```python
from build123d import *

# Parameters (mm, degrees)
BOSS_EXTRUDE1_DEPTH    = 60
CONVERT_SOLID1_DEPTH   = 60
CONVERT_SOLID1_2_DEPTH = 60
SKETCH7_R              = 2
CUT_EXTRUDE2_DEPTH     = 60
SKETCH10_R             = 4.5
CUT_EXTRUDE3_DEPTH     = 10
SKETCH12_R             = 2.5
CUT_EXTRUDE4_DEPTH     = 10


# Read off the part's stored shape, not the designer's step: Convert-Solid1
with BuildPart() as part:
    # Sketch2 → Boss-Extrude1 (new body)
    with BuildSketch(Plane(origin=(0, 0, 0), x_dir=(0, 0, -1), z_dir=(1, 0, 0))):
        Polygon((0, 70), (0, 0), (50, 0), (50, 4), (4, 4), (4, 70), align=None)
    extrude(amount=BOSS_EXTRUDE1_DEPTH)

    # Convert-Solid1 outline → Convert-Solid1 (cut)
    with BuildSketch(Plane.YZ):
        with BuildLine():
            ThreePointArc((0, -8), (2.343145751, -2.343145751), (8, 0))
            Line((8, 0), (0, 0))
            Line((0, 0), (0, -8))
        make_face()
    extrude(amount=CONVERT_SOLID1_DEPTH, mode=Mode.SUBTRACT)

    # Convert-Solid1 2 outline → Convert-Solid1 2 (add)
    with BuildSketch(Plane.YZ):
        with BuildLine():
            ThreePointArc((4, -8), (5.171572875, -5.171572875), (8, -4))
            Line((8, -4), (4, -4))
            Line((4, -4), (4, -8))
        make_face()
    extrude(amount=CONVERT_SOLID1_2_DEPTH)

    # Sketch7 → Cut-Extrude2 (cut)
    with BuildSketch(Plane(origin=(0, 4, 0), x_dir=(1, 0, 0), z_dir=(0, 1, 0))):
        with Locations(Location((15, 29.476677551, 0), (0, 0, 270))):
            Circle(SKETCH7_R)
    cut_extrude2 = extrude(amount=-CUT_EXTRUDE2_DEPTH, mode=Mode.SUBTRACT)

    # Mirror1: Cut-Extrude2 across plane
    add(cut_extrude2.mirror(Plane.ZY.offset(-30)), mode=Mode.SUBTRACT)

    # Sketch10 → Cut-Extrude3 (cut)
    with BuildSketch(Plane(origin=(0, 0, -4), x_dir=(-1, 0, 0), z_dir=(0, 0, -1))):
        with Locations(Location((-30, 32, 0), (0, 0, 90))):
            Circle(SKETCH10_R)
    extrude(amount=-CUT_EXTRUDE3_DEPTH, mode=Mode.SUBTRACT)

    # Sketch12 → Cut-Extrude4 (cut)
    with BuildSketch(Plane(origin=(0, 0, -4), x_dir=(-1, 0, 0), z_dir=(0, 0, -1))):
        with Locations(Location((-48.499902666, 32.060011256, 0), (0, 0, 90))):
            Circle(SKETCH12_R)
        with Locations(Location((-11.5, 32.060011256, 0), (0, 0, 90))):
            Circle(SKETCH12_R)
    extrude(amount=-CUT_EXTRUDE4_DEPTH, mode=Mode.SUBTRACT)


solid = part.part
```
Work out the finished part from the listing and answer in its coordinate system (mm). A direction names the side the tool comes from. Coordinates: 2 decimals unless noted, no trailing zeros. Loops run counter-clockwise (first coordinate to the right, second up) from the corner with the lowest first, then second, coordinate; pieces in that order, holes last. Notation, with made-up numbers: (-3, 81.25) -> (46, 81.25) arc R22 ccw to (46, 113.25) -> close; hole circle Ø10 at (18.25, 31). An arc over 180 degrees is marked (long way). Answer as CSV lines item,"result".
Q1. Find the intervals of material crossed by probe 1 along X at (y, z) = (32, -2.05); probe 2 along Z at (x, y) = (32.5, 40); probe 3 along Y at (x, z) = (52, -38), in increasing order.
Findings:
probe 1,"x = 0 to 9, 14 to 25.5, 34.5 to 46, 51 to 60"
probe 2,"z = -4 to 0"
probe 3,"y = 0 to 4"
Q2. Each of these flat-tipped pins is pushed along its axis until it touches: pin 1 (5 mm diameter, centred on x = 12, y = 16.5, fed in from -Z); pin 2 (3 mm diameter, centred on x = 48.5, y = 32.06, fed in from +Z); pin 3 (8 mm diameter, centred on x = 29.5, z = -15.5, fed in from +Y). Where does it stop, or does it pass through?
Findings:
pin 1,"stops at z = -4"
pin 2,"passes through"
pin 3,"stops at y = 4"
Q3. For a pull along X with two mould halves and no side action, classify faces 1 (the face through (46.774, 2.028, -28.554)), 2 (the face through (30, 70, -2)), 3 (the face through (0, 19, -3)) as +X half, -X half, draft (parallel to the pull), parting line (faces both ways), or undercut.
Findings:
face 1,"undercut"
face 2,"draft"
face 3,"-X half"
Q4. The part is cut by section B-B on y = 32. Write down the section's boundary in (x, z), and give its area (3 significant figures).
Findings:
outline,"(0, -4) -> (9, -4) -> (9, 0) -> (0, 0) -> close; (14, -4) -> (25.5, -4) -> (25.5, 0) -> (14, 0) -> close; (34.5, -4) -> (46, -4) -> (46, 0) -> (34.5, 0) -> close; (51, -4) -> (60, -4) -> (60, 0) -> (51, 0) -> close"
area,"164 mm²"
Q5. The part is cut by section D-D on z = -3. Write down the section's boundary in (x, y) (3 decimals), and give its area (3 significant figures).
Findings:
outline,"(0, 1.755) -> (60, 1.755) -> (60, 70) -> (0, 70) -> close; hole circle Ø5 at (11.5, 32.06); hole circle Ø9 at (30, 32); hole circle Ø5 at (48.5, 32.06)"
area,"3,990 mm²"
Q6. The part is cut by section A-A on x = 11.5. Write down the section's boundary in (y, z), and give its area (3 significant figures).
Findings:
outline,"(0, -50) -> (4, -50) -> (4, -8) arc R4 cw to (8, -4) -> (29.56, -4) -> (29.56, 0) -> (8, 0) arc R8 ccw to (0, -8) -> close; (34.56, -4) -> (70, -4) -> (70, 0) -> (34.56, 0) -> close"
area,"434 mm²"
Q7. A tool of negligible diameter and unlimited length cuts with its end or side. For faces 4 (the face through (16.686, 2.028, -28.401)), 5 (the face through (30, 4, -29)), from which of +Z, -Z, +X, -X, +Y, -Y can it reach the whole face along a straight path? Write none if from no direction.
Findings:
face 4,"+Y, -Y"
face 5,"-Z, +X, -X, +Y"
Q8. The part is cut by section C-C on x = 30. Write down the section's boundary in (y, z).
Findings:
outline,"(0, -50) -> (4, -50) -> (4, -8) arc R4 cw to (8, -4) -> (27.5, -4) -> (27.5, 0) -> (8, 0) arc R8 ccw to (0, -8) -> close; (36.5, -4) -> (70, -4) -> (70, 0) -> (36.5, 0) -> close"
